```python
from build123d import *

# Parameters (mm, degrees)
F0_W     = 76.2
F0_H     = 50.8
F1_DEPTH = 6.35
F2_W     = 76.2
F2_H     = 38.1
F3_DEPTH = 38.1
F5_DEPTH = 38.1
F7_DEPTH = 76.201
F9_DEPTH = 50.801


with BuildPart() as f1:
    # F0 (on Front) → F1 (new body, symmetric)
    with BuildSketch(Plane.XZ):
        with Locations((38.1, 25.4)):
            Rectangle(F0_W, F0_H)
    extrude(amount=F1_DEPTH, both=True)

    # F2 (on face) → F3 (join)
    with BuildSketch(Plane.XZ.offset(6.35)):
        with Locations((38.1, 19.05)):
            Rectangle(F2_W, F2_H)
    extrude(amount=F3_DEPTH)

    # F4 (on face) → F5 (cut)
    with BuildSketch(Plane.XZ.offset(44.45)):
        Polygon((0, 38.1), (0, 0), (38.1, 38.1), align=None)
        Polygon((76.2, 38.1), (38.1, 38.1), (76.2, 0), align=None)
    extrude(amount=-F5_DEPTH, mode=Mode.SUBTRACT)

    # F6 (on Right) → F7 (cut, through all)
    with BuildSketch(Plane.YZ):
        Polygon((-44.45, 0), (-6.35, 38.1), (-44.45, 38.1), align=None)
    extrude(amount=F7_DEPTH, mode=Mode.SUBTRACT)

    # F8 (on face) → F9 (cut, through all)
    with BuildSketch(Plane(origin=(0, 6.35, 0), x_dir=(-1, 0, 0), z_dir=(0, 1, 0))):
        Polygon((0, 50.8), (-25.4, 50.8), (0, 25.4), align=None)
        Polygon((-76.2, 50.8), (-76.2, 25.4), (-50.8, 50.8), align=None)
        Polygon((-57.15, 12.7), (-57.15, 0), (-38.1, 0), (-19.05, 0), (-19.05, 12.7), (-38.1, 12.7), align=None)
    extrude(amount=-F9_DEPTH, mode=Mode.SUBTRACT)


solid = f1.part
```
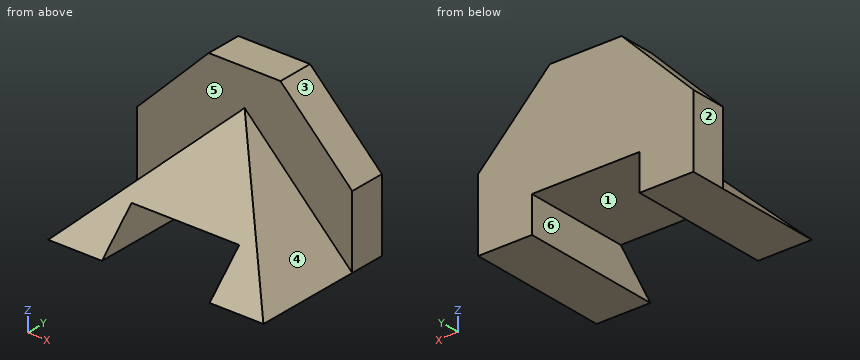
Work out the finished part from the listing and answer in its coordinate system (mm). Face numbers are marked on the shaded views. A direction names the side the tool comes from. Round coordinates to 2 decimals unless told otherwise and drop trailing zeros. Write each loop counter-clockwise with the first axis right and the second up, starting at its lowest first coordinate (ties: lowest second). Pieces come first, ordered by that corner, then holes.
1) A cutting plane is placed at C-C on y = -1. Determine the outline of the cut face in (x, z).
2) Which of the six approach directions +Z, -Z, +X, -X, +Y, -Y give full straight-line access (tool end or side, diameter ignored) to the marked faces 4, 5 and 6?
3) Consider probe 1 along X at (y, z) = (-2.5, 4.5); probe 2 along Y at (x, z) = (14, 15); probe 3 along X at (y, z) = (-30, 5.5). Determine where each line is inside the solid, lowest interval first.
4) A cutting plane is placed at D-D on x = 47. Determine the outline of the cut face in (y, z), and give its area (3 significant figures).
5) Flat-ended cylindrical pins translate along their axes: P1, Ø11.5, axis at x = 30, y = -9, coming from the -Z side; P2, Ø3, axis at x = 23, z = 9.5, coming from the +Y side; P3, Ø15, axis at x = 43, z = 29.5, coming from the -Y side; P4, Ø2, axis at x = 10, z = 29, coming from the -Y side. Find the tip coordinate at first contact, or state that the pin passes through.
6) Determine the mould class of the marked faces 1, 2 and 3 for opening direction X: pulls with the +X half, pulls with the -X half, needs draft (parallel to the pull), parting line crosses it, or undercut.
7) A cutting plane is placed at B-B on y = -41. Determine the outline of the cut face in (x, z).
8) A cutting plane is placed at A-A on z = 4. Determine the outline of the cut face in (x, y).
Entries:
1. outline: (0, 0) - (19.05, 0) - (19.05, 12.7) - (57.15, 12.7) - (57.15, 0) - (76.2, 0) - (76.2, 25.4) - (50.8, 50.8) - (25.4, 50.8) - (0, 25.4) - close
2. face 4: +Z, +X, -Y
2. face 5: +Z, -Y
2. face 6: -Z, +Y, -Y
3. probe 1: x = 0 to 19.05, 57.15 to 76.2
3. probe 2: y = -6.35 to 6.35
3. probe 3: x = 5.5 to 19.05, 57.15 to 70.7
4. outline: (-31.75, 12.7) - (6.35, 12.7) - (6.35, 50.8) - (-6.35, 50.8) - (-6.35, 29.2) - (-15.25, 29.2) - close
4. area: 767 mm2
5. P1: stops at z = 12.7
5. P2: passes through
5. P3: stops at y = -22.45
5. P4: stops at y = -6.35
6. face 1: undercut
6. face 2: pulls with the -X half
6. face 3: pulls with the +X half
7. outline: (0, 0) - (19.05, 0) - (19.05, 3.45) - (3.45, 3.45) - close; (57.15, 0) - (76.2, 0) - (72.75, 3.45) - (57.15, 3.45) - close
8. outline: (0, -6.35) - (4, -6.35) - (4, -40.45) - (19.05, -40.45) - (19.05, 6.35) - (0, 6.35) - close; (57.15, -40.45) - (72.2, -40.45) - (72.2, -6.35) - (76.2, -6.35) - (76.2, 6.35) - (57.15, 6.35) - close
